```python
from build123d import *

# Parameters (mm, degrees)
F0_R     = 28.575
F0_R_2   = 25.4
F0_R_3   = 31.75
F3_DEPTH = 25.4
F4_DEPTH = 5.08
F5_R     = 28.575
F5_R_2   = 25.4
F6_DEPTH = 5.08
F5_R_3   = 31.75
F7_DEPTH = 20.32


# Not quite as in the source:
# - a fillet or chamfer that OpenCascade refuses, or shapes differently, is made with other operations: its cross-section is extruded or revolved along the edge and cut away or added


with BuildPart() as f2:
    # F2: sweep along a path in F1
    with BuildLine(Plane.XY) as f2_path:
        ThreePointArc((76.2, 76.2), (22.3184632736, 53.8815367264), (0, 0))
    # F0 (on Front) → F2 (sweep)
    with BuildSketch(Plane.XZ):
        Circle(F0_R)
        Circle(F0_R_2, mode=Mode.SUBTRACT)
    sweep(path=f2_path.line)

    # F0 (on Front) → F3 (join)
    with BuildSketch(Plane.XZ):
        Circle(F0_R_3)
        Circle(F0_R, mode=Mode.SUBTRACT)
    extrude(amount=F3_DEPTH)

    # F0 (on Front) → F4 (join)
    with BuildSketch(Plane.XZ):
        Circle(F0_R)
        Circle(F0_R_2, mode=Mode.SUBTRACT)
    extrude(amount=F4_DEPTH)

    # F5 (on face) → F6 (join)
    with BuildSketch(Plane.YZ.offset(76.2)):
        with Locations((76.2, 0)):
            Circle(F5_R)
        with Locations((76.2, 0)):
            Circle(F5_R_2, mode=Mode.SUBTRACT)
    extrude(amount=F6_DEPTH)

    # F5 (on face) → F7 (join)
    with BuildSketch(Plane.YZ.offset(76.2)):
        with Locations((76.2, 0)):
            Circle(F5_R_3)
        with Locations((76.2, 0)):
            Circle(F5_R, mode=Mode.SUBTRACT)
    extrude(amount=F7_DEPTH)

    # F8: fillet of radius 5.08 on 4 edges, made by hand

    # F8_s1 → F8_t2 (revolve, cut)
    with BuildSketch(Plane.XY):
        with BuildLine():
            ThreePointArc((76.5707139607, 101.6), (79.4105202921, 102.4678865162), (81.28, 104.775))
            Line((81.28, 104.775), (81.28, 101.6))
            Line((81.28, 101.6), (76.5707139607, 101.6))
        make_face()
    revolve(axis=Axis((81.28, 76.2, 0), (1, 0, 0)), mode=Mode.SUBTRACT)

    # F8_s3 → F8_t4 (revolve, cut)
    with BuildSketch(Plane.XY):
        with BuildLine():
            ThreePointArc((80.9092860393, 107.95), (78.0694797079, 107.0821134838), (76.2, 104.775))
            Line((76.2, 104.775), (76.2, 107.95))
            Line((76.2, 107.95), (80.9092860393, 107.95))
        make_face()
    revolve(axis=Axis((76.2, 76.2, 0), (1, 0, 0)), mode=Mode.SUBTRACT)

    # F8_s5 → F8_t6 (revolve, cut)
    with BuildSketch(Plane.XY):
        with BuildLine():
            ThreePointArc((28.575, -5.08), (26.2678865162, -3.2105202921), (25.4, -0.3707139607))
            Line((25.4, -0.3707139607), (25.4, -5.08))
            Line((25.4, -5.08), (28.575, -5.08))
        make_face()
    revolve(axis=Axis((0, -5.08, 0), (0, -1, 0)), mode=Mode.SUBTRACT)

    # F8_s7 → F8_t8 (revolve, cut)
    with BuildSketch(Plane.XY):
        with BuildLine():
            ThreePointArc((28.575, 0), (30.8821134838, -1.8694797079), (31.75, -4.7092860393))
            Line((31.75, -4.7092860393), (31.75, 0))
            Line((31.75, 0), (28.575, 0))
        make_face()
    revolve(axis=Axis((0, 0, 0), (0, -1, 0)), mode=Mode.SUBTRACT)


solid = f2.part
```
Build history of the part. All positions in model axes, mm. A direction names the side the tool comes from. Coordinates: 2 decimals unless noted, no trailing zeros. Order: outer loops, then holes, each group sorted by start corner. A loop starts at its lowest first (then second) coordinate and runs counter-clockwise, first axis right, second up.
Item 1: Saw through at A-A on z = 0. List the corners of the cut face in (x, y) (3 decimals).
Filled in:
outline: (-31.75, -25.4) - (-28.575, -25.4) - (-28.575, -5.08) arc R5.08 ccw to (-25.4, -0.371) - (-25.4, 0) arc R101.6 cw to (76.2, 101.6) - (76.571, 101.6) arc R5.08 ccw to (81.28, 104.775) - (96.52, 104.775) - (96.52, 107.95) - (80.909, 107.95) arc R5.08 ccw to (76.2, 104.775) arc R104.775 ccw to (-28.575, 0) arc R5.08 ccw to (-31.75, -4.709) - close; (25.4, -0.371) arc R5.08 ccw to (28.575, -5.08) - (28.575, -25.4) - (31.75, -25.4) - (31.75, -4.709) arc R5.08 ccw to (28.575, 0) arc R47.625 cw to (76.2, 47.625) arc R5.08 ccw to (80.909, 44.45) - (96.52, 44.45) - (96.52, 47.625) - (81.28, 47.625) arc R5.08 ccw to (76.571, 50.8) - (76.2, 50.8) arc R50.8 ccw to (25.4, 0) - close
Item 2: Drop flat-ended pins along their axis: pin 1 Ø8 at (x, y) = (74, 65) entering from -Z; pin 2 Ø10 at (y, z) = (67.5, 15) entering from -X; pin 3 Ø4 at (y, z) = (42.5, 16.5) entering from +X. Give the stop position or say it passes through.
Filled in:
pin 1: stops at z = -29.04
pin 2: stops at x = -3.79
pin 3: stops at x = 48.52
Item 3: Tool access for faces 5 (the flat face through (96.52, 50, 12)), 6 (the cylindrical face through (-5.506, -0.183, -24.796)), 7 (the cylindrical face through (88.605, 69.317, -30.995)): list every direction of +Z, -Z, +X, -X, +Y, -Y with a clear straight run to the whole face (end or side of a thin tool).
Filled in:
face 5: +Z, -Z, +X, +Y, -Y
face 6: -Y
face 7: +X
Item 4: Drill centre lines: L1, parallel to Z at x = 91.25, y = 76.2 (3 decimals); L2, parallel to Y at x = 76, z = 0; L3, parallel to Z at x = 11.5, y = 40. Where is each one in solid material? Low to high.
Filled in:
L1: z = -31.75 to -28.575, 28.575 to 31.75
L2: y = 47.62 to 50.8, 101.6 to 104.77
L3: z = -28.57 to -25.4, 25.4 to 28.57
Item 5: Mould opens along Y. For faces 1 (the cylindrical face through (-28.547, -15.098, 1.256)), 2 (the cylindrical face through (88.793, 103.455, 8.583)), 3 (the flat face through (-28.4, -25.4, 4.9)), 4 (the cylindrical face through (76.383, 99.663, -9.728)) say: released by +Y, released by -Y, zero draft, split by the parting line, or undercut.
Filled in:
face 1: zero draft
face 2: undercut
face 3: released by -Y
face 4: undercut
